Check sheet for the modelled part. Datum: model origin and axes. Units: mm. Face numbers are marked on the shaded views. A direction names the side the tool comes from. Coordinates: 2 decimals unless noted, no trailing zeros. Loops run counter-clockwise (first coordinate to the right, second up) from the corner with the lowest first, then second, coordinate; pieces in that order, holes last. Notation, with made-up numbers: (75, -6) - (103, -6) arc R18 cw to (103, 10) - close; hole circle Ø9 at (53.25, 59.5). An arc over 180 degrees is marked (long way). Use a Markdown table: item, result. Add a question column.
1) Sectioned sample at C-C, the plane x = 7.25. Enter the section's corners in (y, z), then the cut area to 3 significant figures.
2) Sectioned sample at D-D, the plane z = 6.35. State how many separate pieces and enclosed holes the cut face has, then the cut area to 3 significant figures.
3) Sectioned sample at B-B, the plane x = 2. Enter the section's corners in (y, z).
4) Tool access check on the marked faces 4, 5 and 6. Record the directions out of +Z, -Z, +X, -X, +Y, -Y that give a thin tool (end or side, any length) a straight path to the whole face; none if there is none.
5) Sectioned sample at A-A, the plane y = -25. Enter the section's corners in (x, z).
6) Draft check along Z on the marked faces 1, 2 and 3. Enter one of: pulls with the +Z half, pulls with the -Z half, needs draft (parallel to the pull), parting line crosses it, or undercut.
7) Thickness scan on line 1 (X direction, y = 12.5, z = 10.25); line 2 (Y direction, x = -4.5, z = 8.5); line 3 (Y direction, x = -3.4, z = 6.35). Record the ranges inside material, lowest first.
8) Go/stop test with flat-tipped pins: P1, Ø7.5, axis at x = 0, y = -25, coming from the +Z side; P2, Ø3, axis at y = -14, z = 8, coming from the +X side; P3, Ø4, axis at y = 9.5, z = 7.5, coming from the -X side; P4, Ø6, axis at y = -33, z = 6.5, coming from the -X side. Record where each tip stops, or that it passes through.
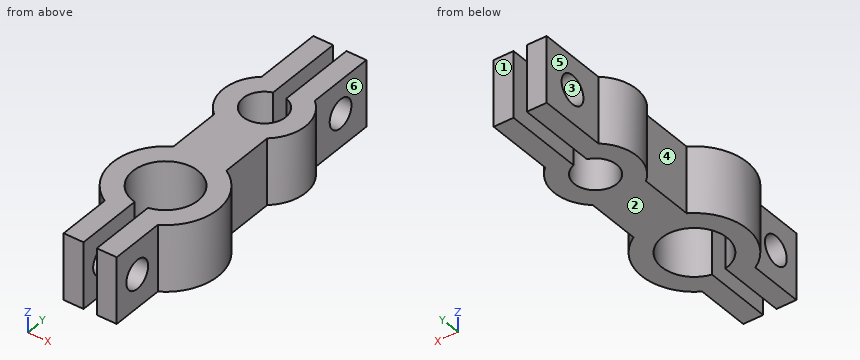
Autodesk Fusion 360 part; units mm, degrees
sketch "Sketch1" plane through (0, 0, 0) normal (0, 0, 1) x (1, 0, 0)
  circle A0 centre (0, 0) radius 4.064
  circle A1 centre (0, 0) radius 7.874
  circle A2 centre (0, -25) radius 10.06
  circle A3 centre (0, -25) radius 6.25
  line L0 (0, 0) -> (0, -25) construction
  line L1 (4.064, 0) -> (-4.064, 0)
  line L2 (-4.064, 0) -> (-4.064, -25)
  line L3 (-4.064, -25) -> (4.064, -25)
  line L4 (4.064, -25) -> (4.064, 0)
  line L5 (4.064, 0) -> (-4.064, -25) construction
  line L6 (-4.064, 0) -> (4.064, -25) construction
  line L7 (-1.27, 19.05) -> (1.27, 19.05)
  line L8 (1.27, 19.05) -> (1.27, -44.05)
  line L9 (1.27, -44.05) -> (-1.27, -44.05)
  line L10 (-1.27, -44.05) -> (-1.27, 19.05)
  line L11 (-1.27, 19.05) -> (1.27, -44.05) construction
  line L12 (1.27, 19.05) -> (-1.27, -44.05) construction
  line L13 (-5.08, 19.05) -> (5.08, 19.05)
  line L14 (5.08, 19.05) -> (5.08, -44.05)
  line L15 (5.08, -44.05) -> (-5.08, -44.05)
  line L16 (-5.08, -44.05) -> (-5.08, 19.05)
  line L17 (-5.08, 19.05) -> (5.08, -44.05) construction
  line L18 (5.08, 19.05) -> (-5.08, -44.05) construction
  point P0 (0, -12.5)
  point P1 (0, -12.5)
  point P2 (0, -12.5)
  dimension "d2" = 3.81
  dimension "d3" = 8.128
  dimension "d4" = 12.5
  dimension "d5" = 3.81
  dimension "d10" = 25
  dimension "d11" = 3.81
  dimension "d13" = 2.54
  dimension "d15" = 19.05
extrude "Extrude1" add sketch "Sketch1" along normal blind 12.7 contours A0 A1 L4 L8 | A0 A1 L4 L8 L14 | A0 A1 L8 L10 | A1 A2 L4 L8 | A1 A2 L4 L14 | A0 A1 L2 L10 L16 | A1 L8 L13 L14 | A0 A1 L2 L10 | A1 A2 L8 L10 | A1 L14 | A2 A3 L4 L8 | A2 A3 L4 L14 | A1 L10 L13 L16 | A1 A2 L2 L10 | A2 A3 L8 L10 | A2 A3 L14 | A1 A2 L2 L16 | A1 L16 | A2 A3 L2 L10 | A2 A3 L2 L16 | A2 L8 L14 L15 | A2 A3 L8 L14 | A2 A3 L16 | A2 A3 L10 L16 | A2 L10 L15 L16 picked at (-0.651, -6.5631) picked at (0.9887, -17.5551)
sketch "Sketch2" plane through (5.08, 0, 0) normal (1, 0, 0) x (0, 1, 0)
  line L0 (-44.05, 0) -> (-33.6832, 0)
  line L1 (-33.6832, 0) -> (-33.6832, 12.7)
  line L2 (-33.6832, 12.7) -> (-44.05, 12.7)
  line L3 (-44.05, 12.7) -> (-44.05, 0)
  line L4 (-38.8666, 12.7) -> (-38.8666, 0)
  point P0 (-38.8666, 6.35)
hole "Hole1" at (5.08, -38.8666, 6.35) direction (-1, 0, 0) diameter 5.5118 depth 40.64 tip angle 180
sketch "Sketch3" plane through (5.08, 0, 0) normal (1, 0, 0) x (0, 1, 0)
  line L0 (6.0161, 0) -> (19.05, 0)
  line L1 (19.05, 0) -> (19.05, 12.7)
  line L2 (19.05, 12.7) -> (6.0161, 12.7)
  line L3 (6.0161, 12.7) -> (6.0161, 0)
  line L4 (12.5331, 12.7) -> (12.5331, 0)
  point P0 (12.5331, 6.35)
hole "Hole2" at (5.08, 12.5331, 6.35) direction (-1, 0, 0) diameter 5.5118 depth 40.64 tip angle 180
Solved:
| question | item | result |
|---|---|---|
| 1 | outline | (-31.97, 0) - (-18.03, 0) - (-18.03, 12.7) - (-31.97, 12.7) - close; (-3.07, 0) - (3.07, 0) - (3.07, 12.7) - (-3.07, 12.7) - close |
| 1 | area | 255 mm2 |
| 2 | separate pieces | 5 |
| 2 | enclosed holes | 0 |
| 2 | area | 481 mm2 |
| 3 | outline | (-44.05, 0) - (-30.92, 0) - (-30.92, 12.7) - (-44.05, 12.7) - close; (-19.08, 0) - (-3.54, 0) - (-3.54, 12.7) - (-19.08, 12.7) - close; (3.54, 0) - (19.05, 0) - (19.05, 12.7) - (3.54, 12.7) - close; hole circle Ø5.51 at (-38.87, 6.35); hole circle Ø5.51 at (12.53, 6.35) |
| 4 | face 4 | +Z, -Z, -X |
| 4 | face 5 | +Z, -Z, -X, +Y |
| 4 | face 6 | +Z, -Z, +X, +Y |
| 5 | outline | (-10.06, 0) - (-6.25, 0) - (-6.25, 12.7) - (-10.06, 12.7) - close; (6.25, 0) - (10.06, 0) - (10.06, 12.7) - (6.25, 12.7) - close |
| 6 | face 1 | needs draft |
| 6 | face 2 | pulls with the -Z half |
| 6 | face 3 | undercut |
| 7 | line 1 | x = -5.08 to -1.27, 1.27 to 5.08 |
| 7 | line 2 | y = -44.05 to -40.59, -37.14 to -29.34, -20.66 to 10.81, 14.26 to 19.05 |
| 7 | line 3 | y = -44.05 to -41.62, -36.11 to -30.24, -19.76 to -2.23, 2.23 to 9.78, 15.29 to 19.05 |
| 8 | P1 | passes through |
| 8 | P2 | stops at x = 5.08 |
| 8 | P3 | stops at x = -5.08 |
| 8 | P4 | stops at x = -8.73 |
